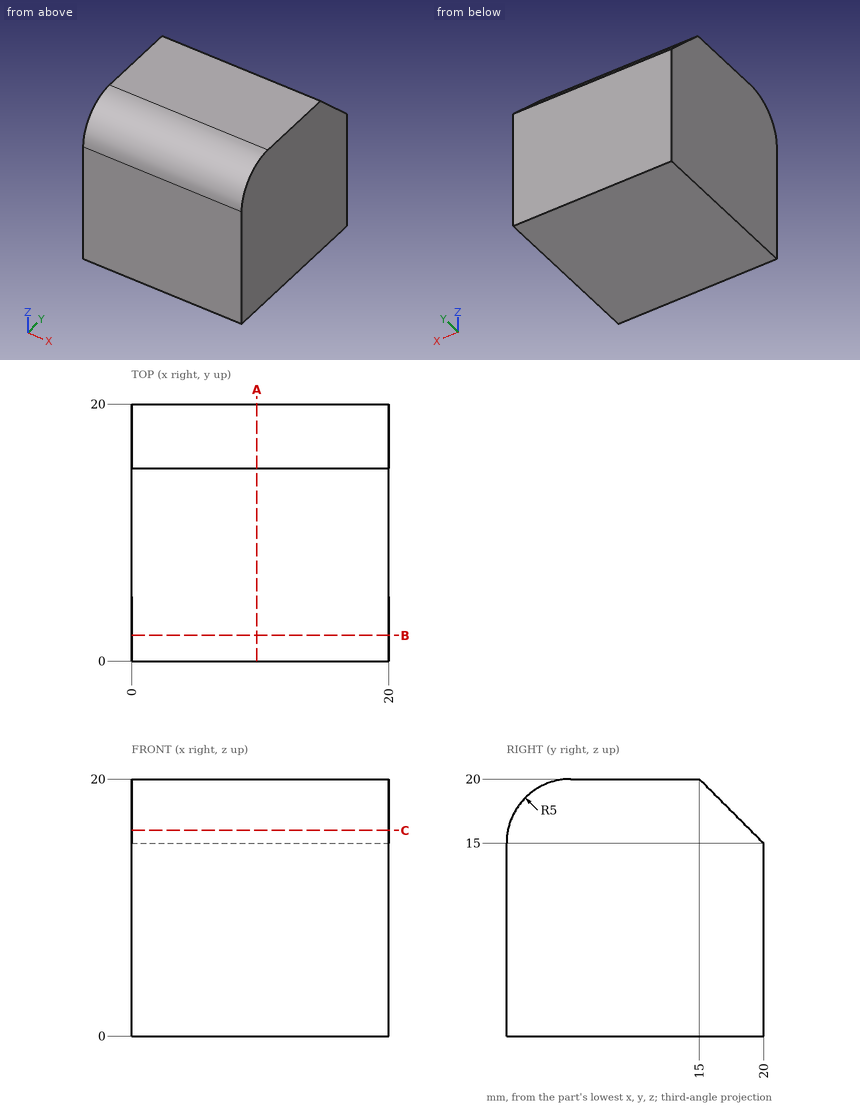
Geometry: see drawing. Coordinates: mm, zero at the bounding-box minimum. Coordinates: 2 decimals unless noted, no trailing zeros. Loops run counter-clockwise (first coordinate to the right, second up) from the corner with the lowest first, then second, coordinate; pieces in that order, holes last.
Q1. Cut plane B-B (y = 2). Output: boundary loops of the cut face in (x, z), then the cut area to 3 significant figures.
Q2. Material intervals for line 1 (Z direction, x = 4, y = 3.25); line 2 (Y direction, x = 4, z = 16); line 3 (Z direction, x = 10.5, y = 3.75), sorted ascending.
Q3. Cut plane C-C (z = 16). Output: boundary loops of the cut face in (x, y), then the cut area to 3 significant figures.
Q4. Cut plane A-A (x = 9.75). Output: boundary loops of the cut face in (y, z).
Working result:
1. outline: (0, 0) - (20, 0) - (20, 19) - (0, 19) - close
1. area: 380 mm2
2. line 1: z = 0 to 19.68
2. line 2: y = 0.1 to 19
2. line 3: z = 0 to 19.84
3. outline: (0, 0.1) - (20, 0.1) - (20, 19) - (0, 19) - close
3. area: 378 mm2
4. outline: (0, 0) - (20, 0) - (20, 15) - (15, 20) - (5, 20) arc R5 ccw to (0, 15) - close
